Could you check a few things on this model? Use its own coordinates, in mm. Face numbers are marked on the shaded views. A direction names the side the tool comes from. Round coordinates to 2 decimals unless told otherwise and drop trailing zeros. Write each loop counter-clockwise with the first axis right and the second up, starting at its lowest first coordinate (ties: lowest second). Pieces come first, ordered by that corner, then holes. Notation, with made-up numbers: (-11.75, 5.5) -> (-6.75, 5.5) arc R13 cw to (-6.75, 17.5) -> close; hole circle Ø10 at (87.5, -36). An arc over 180 degrees is marked (long way). Return JSON: item names as keys, results as strings.
from build123d import *

# Parameters (mm, degrees)
SKETCH2_W          = 38.1
SKETCH2_H          = 6.35
FILLET1_R          = 10
CUT_EXTRUDE1_REACH = 284.088
SKETCH3_R          = 3.175


# Read off the part's stored shape, not the designer's step: Mirror1
with BuildPart() as part:
    # Sweep1: sweep along a path in Sketch1
    with BuildLine(Plane.XY) as sweep1_path:
        Line((0, 0), (38.1, 0))
        Line((38.1, 0), (38.1, 237.998))
        Line((38.1, 237.998), (146.558, 237.998))
    # Sketch2 → Sweep1 (sweep)
    with BuildSketch(Plane(origin=(0, 0, 0), x_dir=(0, 0, -1), z_dir=(1, 0, 0))):
        with Locations((19.05, 3.175)):
            Rectangle(SKETCH2_W, SKETCH2_H)
    sweep(path=sweep1_path.line, transition=Transition.RIGHT)

    # Fillet1
    fillet1_edges = [part.edges().sort_by_distance(p)[0] for p in [
        (31.75, 6.35, -19.05),
        (31.75, 244.348, -19.05),
    ]]
    fillet(fillet1_edges, radius=FILLET1_R)

    # Sketch3 → Cut-Extrude1 (cut, up to next)
    with BuildSketch(Plane(origin=(0, 6.35, 0), x_dir=(1, 0, 0), z_dir=(0, 1, 0)), mode=Mode.PRIVATE) as cut_extrude1_sk1:
        with Locations(Location((10.875, 28.575, 0), (0, 0, 270))):
            Circle(SKETCH3_R)
    cut_extrude1_tool1 = extrude(cut_extrude1_sk1.sketch, amount=-CUT_EXTRUDE1_REACH, mode=Mode.PRIVATE) & part.part
    # Sketch3 → Cut-Extrude1 (cut, up to next)
    with BuildSketch(Plane(origin=(0, 6.35, 0), x_dir=(1, 0, 0), z_dir=(0, 1, 0)), mode=Mode.PRIVATE) as cut_extrude1_sk2:
        with Locations(Location((10.875, 9.525, 0), (0, 0, 270))):
            Circle(SKETCH3_R)
    cut_extrude1_tool2 = extrude(cut_extrude1_sk2.sketch, amount=-CUT_EXTRUDE1_REACH, mode=Mode.PRIVATE) & part.part
    add(cut_extrude1_tool1.solids().sort_by_distance((10.875, 6.35, -28.575))[0], mode=Mode.SUBTRACT)
    add(cut_extrude1_tool2.solids().sort_by_distance((10.875, 6.35, -9.525))[0], mode=Mode.SUBTRACT)

    # Mirror1: part across plane


with BuildPart() as part_1:
    add(part.part)
    add(part.part.mirror(Plane(origin=(146.558, 237.998, 0), x_dir=(0, 0, 1), z_dir=(-1, 0, 0))))


solid = part_1.part
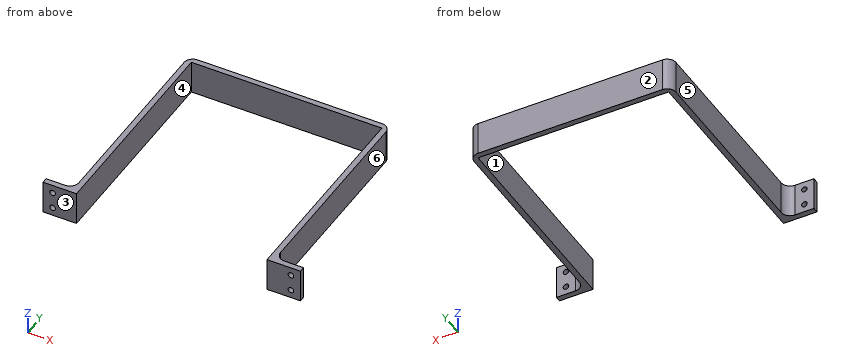
1) I want a section at C-C, the plane x = 98.5. Please give me the cut outline in (y, z), and give its area (3 significant figures).
Return value:
{"outline": "(238, -38.1) -> (244.35, -38.1) -> (244.35, 0) -> (238, 0) -> close", "area": "242 mm²"}
2) Will these pins go through, and if not, where does the flat tip stop? pin 1 Ø2 at (y, z) = (190, -33.5) entering from -X; pin 2 Ø10 at (x, z) = (10.875, -9.525) entering from +Y; pin 3 Ø6 at (x, z) = (89, -20) entering from -Y.
Return value:
{"pin 1": "x = 31.75", "pin 2": "y = 6.35", "pin 3": "y = 238"}
3) I want a section at B-B, the plane z = -18.5. Please give me the cut outline in (x, y).
Return value:
{"outline": "(0, 0) -> (38.1, 0) -> (38.1, 238) -> (255.02, 238) -> (255.02, 0) -> (293.12, 0) -> (293.12, 6.35) -> (271.37, 6.35) arc R10 cw to (261.37, 16.35) -> (261.37, 234.35) arc R10 ccw to (251.37, 244.35) -> (41.75, 244.35) arc R10 ccw to (31.75, 234.35) -> (31.75, 16.35) arc R10 cw to (21.75, 6.35) -> (0, 6.35) -> close"}
4) For the marked faces 1 and 2, which set-ups out of +Z, -Z, +X, -X, +Y, -Y let a thin tool reach every point of the face, with its end or its side?
Return value:
{"face 1": "+Z, -Z, -Y", "face 2": "+Z, -Z, +X, -X, +Y"}
5) I want a section at A-A, the plane y = 213. Please give me the cut outline in (x, z).
Return value:
{"outline": "(31.75, -38.1) -> (38.1, -38.1) -> (38.1, 0) -> (31.75, 0) -> close; (255.02, -38.1) -> (261.37, -38.1) -> (261.37, 0) -> (255.02, 0) -> close"}
6) If I drill on probe 1 along X at (y, z) = (182.5, -7.5); probe 2 along Y at (x, z) = (85, -30); probe 3 along Y at (x, z) = (258, -30.5), over which ranges is the centre line in solid material (lowest first)? Write a range as [from, to].
Return value:
{"probe 1": "[31.75, 38.1], [255.02, 261.37]", "probe 2": "[238, 244.35]", "probe 3": "[0, 241.83]"}
7) Thinking about a two-plate mould opening in X: for the marked faces 3, 4, 5 and 6, which applies, pulls with the +X half, pulls with the -X half, needs draft (parallel to the pull), parting line crosses it, or undercut?
Return value:
{"face 3": "needs draft", "face 4": "undercut", "face 5": "pulls with the -X half", "face 6": "pulls with the +X half"}
